Autodesk Inventor part; units mm, degrees
ref_plane "C1_XY" through (0, 0, 0) normal (0, 0, 1) x (1, 0, 0)
ref_plane "C1_YZ" through (0, 0, 0) normal (1, 0, 0) x (0, 1, 0)
ref_plane "C1_ZX" through (0, 0, 0) normal (0, 1, 0) x (0, 0, 1)
sketch "Sketch_64" plane through (0, 0, 0) normal (0, 0, 1) x (1, 0, 0)
  line L0 (-10, -3) -> (-10, -9)
  arc A0 (-10, -9) -> (-9, -10) centre (-9, -9) ccw
  line L1 (-9, -10) -> (9, -10)
  arc A1 (9, -10) -> (10, -9) centre (9, -9) ccw
  line L2 (10, -9) -> (10, 9)
  arc A2 (10, 9) -> (9, 10) centre (9, 9) ccw
  line L3 (9, 10) -> (3, 10)
  line L4 (3, 10) -> (3, 8)
  line L5 (3, 8) -> (6, 8)
  line L6 (6, 8) -> (6, 7.0607)
  line L7 (6, 7.0607) -> (2.9393, 4)
  line L8 (2.9393, 4) -> (0.5196, 4)
  line L9 (0.5196, 4) -> (0, 3.7)
  line L10 (0, 3.7) -> (-0.5196, 4)
  line L11 (-0.5196, 4) -> (-2.9393, 4)
  line L12 (-2.9393, 4) -> (-6, 7.0607)
  line L13 (-6, 7.0607) -> (-6, 8)
  line L14 (-6, 8) -> (-3, 8)
  line L15 (-3, 8) -> (-3, 10)
  line L16 (-3, 10) -> (-9, 10)
  arc A3 (-9, 10) -> (-10, 9) centre (-9, 9) ccw
  line L17 (-10, 9) -> (-10, 3)
  line L18 (-10, 3) -> (-8, 3)
  line L19 (-8, 3) -> (-8, 6)
  line L20 (-8, 6) -> (-7.0607, 6)
  line L21 (-7.0607, 6) -> (-4, 2.9393)
  line L22 (-4, 2.9393) -> (-4, 0.5196)
  line L23 (-4, 0.5196) -> (-3.7, 0)
  line L24 (-3.7, 0) -> (-4, -0.5196)
  line L25 (-4, -0.5196) -> (-4, -2.9393)
  line L26 (-4, -2.9393) -> (-7.0607, -6)
  line L27 (-7.0607, -6) -> (-8, -6)
  line L28 (-8, -6) -> (-8, -3)
  line L29 (-8, -3) -> (-10, -3)
  line L30 (-6, -7.2678) -> (-6, -7.5)
  arc A4 (-6, -7.5) -> (-5.5, -8) centre (-5.5, -7.5) ccw
  line L31 (-5.5, -8) -> (7, -8)
  arc A5 (7, -8) -> (8, -7) centre (7, -7) ccw
  line L32 (8, -7) -> (8, 5.5)
  arc A6 (8, 5.5) -> (7.5, 6) centre (7.5, 5.5) ccw
  line L33 (7.5, 6) -> (7.2678, 6)
  arc A7 (7.2678, 6) -> (6.9142, 5.8536) centre (7.2678, 5.5) ccw
  line L34 (6.9142, 5.8536) -> (4.1464, 3.0858)
  arc A8 (4.1464, 3.0858) -> (4, 2.7322) centre (4.5, 2.7322) ccw
  line L35 (4, 2.7322) -> (4, -1)
  arc A9 (1, -4) -> (4, -1) centre (1, -1) ccw
  line L36 (1, -4) -> (-2.7322, -4)
  arc A10 (-2.7322, -4) -> (-3.0858, -4.1464) centre (-2.7322, -4.5) ccw
  line L37 (-3.0858, -4.1464) -> (-5.8536, -6.9142)
  arc A11 (-5.8536, -6.9142) -> (-6, -7.2678) centre (-5.5, -7.2678) ccw
extrude "Extrusion1" add sketch "Sketch_64" against normal blind 456
sketch "Sketch2" plane through (0, 0, -456) normal (0, 0, -1) x (-1, 0, 0)
  point P0 (0, 0)
hole "Hole1" at (0, 0, -456) direction (0, 0, 1) diameter 4.2 depth 456
ref_plane "C1_XY" through (0, 0, 0) normal (0, 0, 1) x (1, 0, 0)
ref_plane "C1_YZ" through (0, 0, 0) normal (1, 0, 0) x (0, 1, 0)
ref_plane "C1_ZX" through (0, 0, 0) normal (0, 1, 0) x (0, 0, 1)
thread "Thread1"
thread "Thread2"
properties part number "HFSTB5-2020-456" material "Aluminum 6061"
Part model, mm, in its own coordinate system. A direction names the side the tool comes from. Coordinates: 2 decimals unless noted, no trailing zeros. Use a Markdown table: item, result. Add a question column.
Q1. Pin check, flat tips, straight feed: P1, Ø2.5, axis at y = -1.5, z = -127.5, coming from the -X side; P2, Ø1.9, axis at x = 1.5, z = -117.5, coming from the +Y side; P3, Ø3.5, axis at x = 0, y = 0, coming from the -Z side. Stop position of each tip, or through.
Q2. Cut at A-A (z = -222.5). Give the number of separate pieces and of enclosed holes in the cut face, and give its area (3 significant figures).
Q3. Which spindle directions (+Z, -Z, +X, -X, +Y, -Y) get a long thin tool onto all of the face, cutting with end or side? Do faces 1 (the flat face through (0, -10, -225)), 2 (the flat face through (1, -8, -225)). Say none if no direction does.
Q4. Probe L1, parallel to Y at x = 0, z = -202; L2, parallel to X at y = 0, z = -364.5; L3, parallel to X at y = 8.25, z = -158.5. List the from-to ranges inside material, lowest first.
Q5. Mould opens along X. For faces 3 (the flat face through (-0.1, 2.4, 0)), 4 (the flat face through (10, 0, -225)), 5 (the flat face through (8, -1, -225)) say: +X half, -X half, draft (parallel to the pull), parting line (faces both ways), or undercut.
Worked out:
| question | item | result |
|---|---|---|
| 1 | P1 | stops at x = -4 |
| 1 | P2 | stops at y = 4 |
| 1 | P3 | passes through |
| 2 | separate pieces | 1 |
| 2 | enclosed holes | 2 |
| 2 | area | 195 mm2 |
| 3 | face 1 | +Z, -Z, +X, -X, -Y |
| 3 | face 2 | +Z, -Z |
| 4 | L1 | y = -10 to -8, -4 to -2.1, 2.1 to 3.7 |
| 4 | L2 | x = -3.7 to -2.1, 2.1 to 4, 8 to 10 |
| 4 | L3 | x = -10 to -3, 3 to 10 |
| 5 | face 3 | draft |
| 5 | face 4 | +X half |
| 5 | face 5 | undercut |
